Geometry check sheet. Reference: the model listing, model coordinates, mm. Face numbers are marked on the shaded views. A direction names the side the tool comes from. Round coordinates to 2 decimals unless told otherwise and drop trailing zeros. Order: outer loops, then holes, each group sorted by start corner. A loop starts at its lowest first (then second) coordinate and runs counter-clockwise, first axis right, second up. Notation, with made-up numbers: (-32.75, 38.25) - (-20.75, 38.25) arc R21 ccw to (-20.75, 60.25) - close; hole circle Ø10 at (38.5, 57). An arc over 180 degrees is marked (long way). Return JSON: item names as keys, results as strings. Group by question number.
Q1. Sectioned sample at B-B, the plane z = 12. Give the number of separate pieces and of enclosed holes in the cut face, then the cut area to 3 significant figures.
Q2. Tool access check on the marked faces 1 and 2. Record the directions out of +Z, -Z, +X, -X, +Y, -Y that give a thin tool (end or side, any length) a straight path to the whole face; none if there is none.
Q3. Material ranges on line 1 along X through (y, z) = (0.85, 12); line 2 along Z through (x, y) = (25.5, 6.5); line 3 along X through (y, z) = (0.65, 12), recorded low to high.
Q4. Sectioned sample at A-A, the plane x = 19. Record the cut outline in (y, z), then the cut area to 3 significant figures.
Q5. Sectioned sample at C-C, the plane y = 9. Record the cut outline in (x, z).
Q6. Gauge pin test, flat ends, axial feed: pin 1 Ø2 at (x, z) = (-17.5, -13) entering from +Y; pin 2 Ø0.5 at (y, z) = (13, 14.5) entering from -X; pin 3 Ø1.1 at (y, z) = (7, 14.5) entering from +X. Record the tip position at first contact, or that the pin passes through.
Q7. Draft check along Z on the marked faces 3, 4 and 5. Enter one of: pulls with the +Z half, pulls with the -Z half, needs draft (parallel to the pull), parting line crosses it, or undercut.
```python
from build123d import *

# Parameters (mm, degrees)
SKETCH1_W           = 67
SKETCH1_H           = 34
BOSS_EXTRUDE1_DEPTH = 20
SKETCH4_W           = 63
SKETCH4_H           = 30
CUT_EXTRUDE1_DEPTH  = 18
SKETCH5_W           = 28
SKETCH5_H           = 18
CUT_EXTRUDE4_DEPTH  = 2
SKETCH8_W           = 28
SKETCH8_H           = 18
CUT_EXTRUDE5_DEPTH  = 2
SKETCH9_R           = 2.5
SKETCH9_R_2         = 2.277231992
CUT_EXTRUDE6_DEPTH  = 2
FILLET1_R           = 1


with BuildPart() as part:
    # Sketch1 → Boss-Extrude1 (new body)
    with BuildSketch(Plane(origin=(0, 0, 0), x_dir=(1, 0, 0), z_dir=(0, 1, 0))):
        Rectangle(SKETCH1_W, SKETCH1_H)
    extrude(amount=BOSS_EXTRUDE1_DEPTH)

    # Sketch4 → Cut-Extrude1 (cut)
    with BuildSketch(Plane(origin=(0, 20, 0), x_dir=(1, 0, 0), z_dir=(0, 1, 0))):
        Rectangle(SKETCH4_W, SKETCH4_H)
    extrude(amount=-CUT_EXTRUDE1_DEPTH, mode=Mode.SUBTRACT)

    # Sketch5 → Cut-Extrude4 (cut)
    with BuildSketch(Plane(origin=(33.5, 0, 0), x_dir=(0, 0, -1), z_dir=(1, 0, 0))):
        with Locations((0, 11)):
            Rectangle(SKETCH5_W, SKETCH5_H)
    extrude(amount=-CUT_EXTRUDE4_DEPTH, mode=Mode.SUBTRACT)

    # Sketch8 → Cut-Extrude5 (cut)
    with BuildSketch(Plane.ZY.offset(33.5)):
        with Locations((0, 11)):
            Rectangle(SKETCH8_W, SKETCH8_H)
    extrude(amount=-CUT_EXTRUDE5_DEPTH, mode=Mode.SUBTRACT)

    # Sketch9 → Cut-Extrude6 (cut)
    with BuildSketch(Plane.XZ):
        with Locations(Location((19, 12, 0), (0, 0, 270))):
            Circle(SKETCH9_R)
        with Locations(Location((19, -12, 0), (0, 0, 90))):
            Circle(SKETCH9_R)
        with Locations(Location((-13.5, 12, 0), (0, 0, 270))):
            Circle(SKETCH9_R_2)
        with Locations(Location((-13.5, -12, 0), (0, 0, 90))):
            Circle(SKETCH9_R_2)
    extrude(amount=-CUT_EXTRUDE6_DEPTH, mode=Mode.SUBTRACT)

    # Fillet1
    fillet1_edges = [part.edges().sort_by_distance(p)[0] for p in [
        (-33.5, 20, -15.5),
        (0, 20, 17),
        (33.5, 20, -15.5),
        (33.5, 11, -14),
        (33.5, 11, 14),
        (33.5, 2, 0),
        (-33.5, 20, 15.5),
        (-33.5, 11, 14),
        (-33.5, 11, -14),
        (-33.5, 2, 0),
        (33.5, 20, 15.5),
        (0, 0, 17),
        (-33.5, 0, 0),
        (0, 0, -17),
        (33.5, 0, 0),
        (33.5, 10, 17),
        (-33.5, 10, 17),
        (-33.5, 10, -17),
        (33.5, 10, -17),
        (0, 20, -17),
    ]]
    fillet(fillet1_edges, radius=FILLET1_R - 0.0001)  # a hair under: the kernel refuses the full size


solid = part.part
```
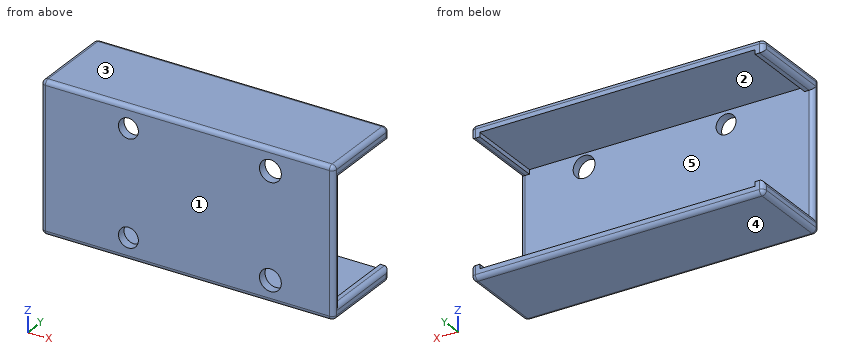
Reply:
{
 "1": {"separate pieces": "3", "enclosed holes": "0", "area": "114 mm^2"},
 "2": {"face 1": "+Z, -Z, +X, -X, -Y", "face 2": "+Y"},
 "3": {"line 1": "-33.49 to -15.78, -11.22 to 16.5, 21.5 to 33.49", "line 2": "-17 to -15, 15 to 17", "line 3": "-33.44 to -15.78, -11.22 to 16.5, 21.5 to 33.44"},
 "4": {"outline": "(0, -16) arc R1 ccw to (1, -17) - (19, -17) arc R1 ccw to (20, -16) - (20, -15) - (2, -15) - (2, -14.5) - (0, -14.5) - close; (0, -9.5) - (2, -9.5) - (2, 9.5) - (0, 9.5) - close; (0, 14.5) - (2, 14.5) - (2, 15) - (20, 15) - (20, 16) arc R1 ccw to (19, 17) - (1, 17) arc R1 ccw to (0, 16) - close", "area": "119 mm^2"},
 "5": {"outline": "(-33.5, -16) arc R1 ccw to (-32.5, -17) - (32.5, -17) arc R1 ccw to (33.5, -16) - (33.5, -15) arc R1 ccw to (32.5, -14) - (31.5, -14) - (31.5, -15) - (-31.5, -15) - (-31.5, -14) - (-32.5, -14) arc R1 ccw to (-33.5, -15) - close; (-33.5, 15) arc R1 ccw to (-32.5, 14) - (-31.5, 14) - (-31.5, 15) - (31.5, 15) - (31.5, 14) - (32.5, 14) arc R1 ccw to (33.5, 15) - (33.5, 16) arc R1 ccw to (32.5, 17) - (-32.5, 17) arc R1 ccw to (-33.5, 16) - close"},
 "6": {"pin 1": "y = 2", "pin 2": "x = -33.47", "pin 3": "x = 33.5"},
 "7": {"face 3": "pulls with the +Z half", "face 4": "pulls with the -Z half", "face 5": "undercut"}
}
